Could you check a few things on this model? Use its own coordinates, in mm. A direction names the side the tool comes from. Coordinates: 2 decimals unless noted, no trailing zeros. Order: outer loops, then holes, each group sorted by start corner. A loop starts at its lowest first (then second) coordinate and runs counter-clockwise, first axis right, second up. Notation, with made-up numbers: M -8,83 L 31,83 A14 ccw 31,89 Z; hole C 70,-26 d7. An arc over 180 degrees is marked long. Put each result on its own line as item: value. Start each with the question number.
```python
from build123d import *

# Parameters (mm, degrees)
BOSS_EXTRUDE1_DEPTH            = 2.4
BOSS_EXTRUDE2_DEPTH            = 2.4
BOSS_EXTRUDE2_DEPTH_BACK       = 2
FILLET1_R                      = 8
FILLET2_R                      = 2
F_3_0MM_START                  = -2
F_3_0MM_DOWEL_SLOT1_DEPTH      = 4.4
F_4_0_4_DIAMETER_HOLE1_D       = 4
CBORE_FOR_M3_SHCS1_D           = 3.4
CBORE_FOR_M3_SHCS1_CBORE_D     = 6.5
CBORE_FOR_M3_SHCS1_CBORE_DEPTH = 2
FILLET5_R                      = 2
FILLET6_R                      = 1
FILLET8_R                      = 2
CUT_EXTRUDE1_DEPTH             = 38
CHAMFER2_SIZE2                 = 1.9
CHAMFER2_SIZE                  = 5.220207097
FILLET9_R                      = 3


# Read off the part's stored shape, not the designer's step: Ø3.0mm Dowel Slot1
# Some blends are built 0.0001 mm under size
with BuildPart() as part:
    # Sketch1 → Boss-Extrude1 (new body)
    with BuildSketch(Plane(origin=(0, 0, 0), x_dir=(1, 0, 0), z_dir=(0, 1, 0))):
        with BuildLine():
            Line((2, 7.720929875), (-51.546411114, 0.671411114))
            ThreePointArc((-51.546411114, 0.671411114), (-51.035673477, -0.364262362), (-50, -0.875))
            Line((-50, -0.875), (20, -10.090674831))
            Line((20, -10.090674831), (20, 8))
            Line((20, 8), (7, 8))
            Line((7, 8), (7, 14))
            Line((7, 14), (2, 14))
            Line((2, 14), (2, 7.720929875))
        make_face()
    extrude(amount=BOSS_EXTRUDE1_DEPTH)

    # Sketch1<6> → Boss-Extrude2 (add, two sides: drawn at the far end of the back side and taken through both)
    with BuildSketch(Plane(origin=(0, 0, 0), x_dir=(1, 0, 0), z_dir=(0, 1, 0)).offset(-BOSS_EXTRUDE2_DEPTH_BACK)):
        with BuildLine():
            Line((20, 8), (20, -10.090674831))
            Line((20, -10.090674831), (20, -19.5))
            Line((20, -19.5), (26, -19.5))
            ThreePointArc((26, -19.5), (31.86887196, -6.373774392), (31.5, 8))
            Line((31.5, 8), (20, 8))
        make_face()
    extrude(amount=BOSS_EXTRUDE2_DEPTH + BOSS_EXTRUDE2_DEPTH_BACK)

    # Fillet1
    fillet1_edges = [part.edges().sort_by_distance(p)[0] for p in [
        (20, 1.2, 10.090674831),
    ]]
    fillet(fillet1_edges, radius=FILLET1_R)

    # Fillet2
    fillet2_edges = [part.edges().sort_by_distance(p)[0] for p in [
        (20, 0.2, 19.5),
        (31.5, 0.2, -8),
        (26, 0.2, 19.5),
    ]]
    fillet(fillet2_edges, radius=FILLET2_R)

    # Ø3.0mm Dowel Slot1 outline → Ø3.0mm Dowel Slot1 (cut)
    with BuildSketch(Plane(origin=(0, 0, 0), x_dir=(1, 0, 0), z_dir=(0, 1, 0)).offset(F_3_0MM_START)):
        with BuildLine():
            Line((26.5, -1.5), (28.5, -1.5))
            ThreePointArc((28.5, -1.5), (30, 0), (28.5, 1.5))
            Line((28.5, 1.5), (26.5, 1.5))
            ThreePointArc((26.5, 1.5), (25, 0), (26.5, -1.5))
        make_face()
    extrude(amount=F_3_0MM_DOWEL_SLOT1_DEPTH, mode=Mode.SUBTRACT)

    # Ø4.0 (4) Diameter Hole1 (through all)
    with Locations(Plane(origin=(0, 2.4, 0), x_dir=(1, 0, 0), z_dir=(0, 1, 0))):
        with Locations((0, 0)):
            Hole(F_4_0_4_DIAMETER_HOLE1_D / 2)

    # CBORE for M3 SHCS1 (through all)
    with Locations(Plane(origin=(0, 2.4, 0), x_dir=(1, 0, 0), z_dir=(0, 1, 0))):
        with Locations((25.841547072, -9.405553941)):
            CounterBoreHole(CBORE_FOR_M3_SHCS1_D / 2, CBORE_FOR_M3_SHCS1_CBORE_D / 2, CBORE_FOR_M3_SHCS1_CBORE_DEPTH)

    # Fillet5
    fillet5_edges = [part.edges().sort_by_distance(p)[0] for p in [
        (2, 1.2, -7.720929875),
        (7, 1.2, -8),
    ]]
    fillet(fillet5_edges, radius=FILLET5_R)

    # Fillet6
    fillet6_edges = [part.edges().sort_by_distance(p)[0] for p in [
        (4.5, 0, -14),
        (2, 1.2, -14),
        (7, 1.2, -14),
        (4.5, 2.4, -14),
    ]]
    fillet(fillet6_edges, radius=FILLET6_R)

    # Chamfer1
    # the kernel refuses this chamfer: 0.5 mm, written as the material it takes off along each edge
    with BuildSketch(Plane(origin=(0, -2, 0), x_dir=(0.7609198459057782, 0, 0.6488458893348455), z_dir=(-0.6488458893348455, 0, 0.7609198459057782))) as chamfer1_piece_1:
        with BuildLine():
            Line((32.514142136, 0.514142136), (31.985857864, -0.014142136))
            Line((31.985857864, -0.014142136), (31.985857864, -0.024142136))
            ThreePointArc((31.985857864, -0.024142136), (32.242928932, -0.01), (32.5, -0.01))
            Line((32.5, -0.01), (32.51, 0))
            ThreePointArc((32.51, 0), (32.51, 0.257071068), (32.524142136, 0.514142136))
            Line((32.524142136, 0.514142136), (32.514142136, 0.514142136))
        make_face()
    revolve(axis=Axis((0, -2, 0), (0, 1, 0)), revolution_arc=57.24100759, mode=Mode.SUBTRACT)

    # Fillet8
    fillet8_edges = [part.edges().sort_by_distance(p)[0] for p in [
        (20, 0, 4.553243268),
    ]]
    fillet(fillet8_edges, radius=FILLET8_R - 0.0001)  # a hair under: the kernel refuses the full size

    # Sketch8 → Cut-Extrude1 (cut)
    with BuildSketch(Plane(origin=(-50.581323439, 0, 6.659157562), x_dir=(0, -1, 0), z_dir=(0.9914448613738104, 0, -0.13052619222005302))):
        Polygon((-1.9, 7.393823865), (0, 2.173616768), (0, 7.393823865), align=None)
    extrude(amount=CUT_EXTRUDE1_DEPTH, mode=Mode.SUBTRACT)

    # Chamfer2
    chamfer2_edges = [part.edges().sort_by_distance(p)[0] for p in [
        (-13.530819505, 0, -3.043632668),
    ]]
    chamfer2_side = [part.faces().sort_by_distance(p)[0] for p in [
        (-13.4931446, 0, -3.048592663),
    ]]
    chamfer(chamfer2_edges, length=CHAMFER2_SIZE - 0.0001, length2=CHAMFER2_SIZE2 - 0.0001, reference=chamfer2_side[0])  # a hair under: the kernel refuses the full size

    # Fillet9
    fillet9_edges = [part.edges().sort_by_distance(p)[0] for p in [
        (-10.943077395, 0.94995, -3.384176821),
    ]]
    fillet(fillet9_edges, radius=FILLET9_R)


solid = part.part
```
Item 1: If we section it at B-B on x = -34: Write out the boundary of the cut face in (y, z), then the cut area to 3 significant figures.
Item 2: If we mould it in two halves opening along X, with no side actions, what happens to faces 1 (the flat face through (25, -2, 6)), 2 (the cylindrical face through (0, 1, 2)), 3 (the conical face through (31.411, -1.865, 6.787)), 4 (the cylindrical face through (19.43, -0.6, 4.38))? For each: released by +X, released by -X, zero draft, split by the parting line, or undercut.
Item 3: For faces 5 (the flat face through (23, 0, 19.5)), 6 (the flat face through (27, 0, 1.5)), 7 (the flat face through (-9.724, 0.435, -4.973)), 8 (the cylindrical face through (31.77, 0.42, 6.85)), 9 (the flat face through (22, 1, -8)), which set-ups out of +Z, -Z, +X, -X, +Y, -Y let a thin tool reach every point of the face, with its end or its side?
Item 4: I need wall thicknesses on probe 1 along Z at (x, y) = (28, -0.45); probe 2 along Y at (x, z) = (16.5, 8); probe 3 along Z at (x, y) = (23, 1.05). Which ranges of each line are inside material? Lowest first, please.
Item 5: For pin 1 Ø2.5 at (x, z) = (25.84, 9.41) entering from -Y; pin 2 Ø0.6 at (x, y) = (27.5, 0) entering from +Z; pin 3 Ø1.5 at (x, z) = (16.5, -0.5) entering from -Y; pin 4 Ø1.6 at (x, y) = (27.5, 1) entering from -Z, each with a flat end and sliding along its axis, tell me the tip position at first contact or that it passes through.
Item 6: If we section it at A-A on x = -25: Write out the boundary of the cut face in (y, z), then the cut area to 3 significant figures.
Geometry check:
1. outline: M 0,2.28 L 1.9,-2.98 L 2.4,-2.98 L 2.4,2.98 L 0,2.98 Z
1. area: 9.31 mm²
2. face 1: zero draft
2. face 2: undercut
2. face 3: released by +X
2. face 4: released by -X
3. face 5: +Z, +X, -X, +Y, -Y
3. face 6: +Y, -Y
3. face 7: -X, -Y
3. face 8: +X, +Y, -Y
3. face 9: -Z, +X, +Y, -Y
4. probe 1: z = -8 to -1.5, 1.5 to 16.5
4. probe 2: y = 0 to 2.4
4. probe 3: z = -8 to 7.83, 10.98 to 19.5
5. pin 1: passes through
5. pin 2: stops at z = 17.79
5. pin 3: stops at y = 0
5. pin 4: stops at z = -8
6. outline: M 0,1.1 L 1.9,-4.17 L 2.4,-4.17 L 2.4,4.17 L 0,4.17 Z
6. area: 15.0 mm²
